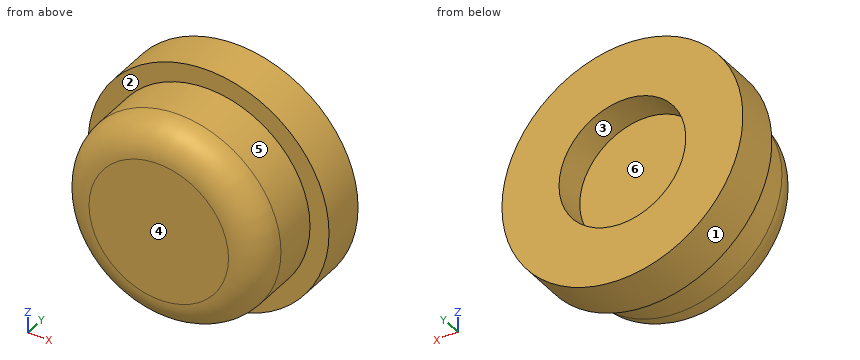
from build123d import *

# Parameters (mm, degrees)
SKETCH046_R     = 3.8
PAD020_DEPTH    = 1.4
SKETCH047_R     = 3.2
PAD021_DEPTH    = 2.4
SKETCH049_R     = 2
POCKET020_DEPTH = 1
FILLET018_R     = 1


with BuildPart() as part:
    # Sketch046 → Pad020 (new body)
    with BuildSketch(Plane.XZ):
        with Locations((28.8, 9.2)):
            Circle(SKETCH046_R)
    extrude(amount=PAD020_DEPTH)

    # Sketch047 (on Face3 of Pad020) → Pad021 (join)
    with BuildSketch(Plane.XZ.offset(1.4)):
        with Locations((28.8, 9.2)):
            Circle(SKETCH047_R)
    extrude(amount=PAD021_DEPTH)

    # Sketch049 (on Face2 of Pad021) → Pocket020 (cut)
    with BuildSketch(Plane(origin=(0, 0, 0), x_dir=(1, 0, 0), z_dir=(0, 1, 0))):
        with Locations((28.8, -9.2)):
            Circle(SKETCH049_R)
    extrude(amount=-POCKET020_DEPTH, mode=Mode.SUBTRACT)

    # Fillet018
    fillet018_edges = [part.edges().sort_by_distance(p)[0] for p in [
        (25.6, -3.8, 9.2),
    ]]
    fillet(fillet018_edges, radius=FILLET018_R)


solid = part.part
Geometry: final body of the model. Coordinates: model frame, mm. Face numbers are marked on the shaded views. A direction names the side the tool comes from. Give positions to 0.01 mm unless a question says otherwise; leave off trailing zeros. Order: outer loops, then holes, each group sorted by start corner. A loop starts at its lowest first (then second) coordinate and runs counter-clockwise, first axis right, second up. Notation, with made-up numbers: (72, -31) -> (126, -31) arc R11 cw to (126, -25) -> close; hole circle Ø3 at (4, 31.5). An arc over 180 degrees is marked (long way). Put each result on its own line as item: value.
Q1. Section D-D, the plane y = -3.5. Return loops of the section in (x, z).
Here are the results:
outline: circle Ø5.83 at (28.8, 9.2)
Q2. Section A-A, the plane x = 28.8. Return loops of the section in (y, z).
Here are the results:
outline: (-3.8, 7) arc R1 ccw to (-2.8, 6) -> (-1.4, 6) -> (-1.4, 5.4) -> (0, 5.4) -> (0, 7.2) -> (-1, 7.2) -> (-1, 11.2) -> (0, 11.2) -> (0, 13) -> (-1.4, 13) -> (-1.4, 12.4) -> (-2.8, 12.4) arc R1 ccw to (-3.8, 11.4) -> close
Q3. Draft query along X for the marked faces 4, 5 and 6. Return one class per face: released by +X, released by -X, zero draft, split by the parting line, or undercut.
Here are the results:
face 4: zero draft
face 5: split by the parting line
face 6: undercut
Q4. Section C-C, the plane y = -2.6. Return loops of the section in (x, z).
Here are the results:
outline: circle Ø6.4 at (28.8, 9.2)
Q5. Material intervals for L1, parallel to Z at x = 28.8, y = -0.3; L2, parallel to Y at x = 26.5, z = 6.75; L3, parallel to Y at x = 29.25, z = 10.75, sorted ascending.
Here are the results:
L1: z = 5.4 to 7.2, 11.2 to 13
L2: y = -1.4 to 0
L3: y = -3.8 to -1
Q6. Reachability of the marked faces 1, 2 and 3 from +Z, -Z, +X, -X, +Y, -Y: full face, straight path, thin tool, end or side. Return the list, or none.
Here are the results:
face 1: +Y, -Y
face 2: -Y
face 3: +Y
Q7. Pin query (flat end, axial travel): pin 1 (1.5 mm diameter, centred on x = 30, y = -3, fed in from +Z); pin 2 (1 mm diameter, centred on x = 30.5, y = -2.5, fed in from -Z). Return the tip coordinate at first contact, or that it passes through.
Here are the results:
pin 1: stops at z = 12.36
pin 2: stops at z = 6.23
Q8. Section B-B, the plane z = 9.2. Return loops of the section in (x, y).
Here are the results:
outline: (25, -1.4) -> (25.6, -1.4) -> (25.6, -2.8) arc R1 ccw to (26.6, -3.8) -> (31, -3.8) arc R1 ccw to (32, -2.8) -> (32, -1.4) -> (32.6, -1.4) -> (32.6, 0) -> (30.8, 0) -> (30.8, -1) -> (26.8, -1) -> (26.8, 0) -> (25, 0) -> close
